Read the model definition and answer for the solid it produces. Units are mm, in the model's axes. Face numbers are marked on the shaded views. A direction names the side the tool comes from. Coordinates: 2 decimals unless noted, no trailing zeros. Write each loop counter-clockwise with the first axis right and the second up, starting at its lowest first coordinate (ties: lowest second). Pieces come first, ordered by that corner, then holes. Notation, with made-up numbers: (-0.75, 66) -> (20.25, 66) arc R26 ccw to (20.25, 87) -> close; hole circle Ø11 at (24.5, 5). An arc over 180 degrees is marked (long way). Answer in a Markdown table with one row per item. Add a question column.
Item 1: Given pin 1 Ø1 at (y, z) = (3.5, 31.5) entering from +X; pin 2 Ø4 at (y, z) = (-18, 16.5) entering from -X; pin 3 Ø16 at (x, y) = (-32.7, 0) entering from +Z, each flat-ended and moving along its own axis, determine where each tip first touches the part or whether it passes through.
Item 2: Which of the six approach directions +Z, -Z, +X, -X, +Y, -Y give full straight-line access (tool end or side, diameter ignored) to the marked faces 1 and 2?
Item 3: Section C-C on y = -15.5 is taken. Write down the section's boundary in (x, z), then the cut area to 3 significant figures.
Item 4: Section A-A on z = 5.5 is taken. Write down the section's boundary in (x, y), then the cut area to 3 significant figures.
Item 5: Section B-B on x = 12.5 is taken. Write down the section's boundary in (y, z).
Item 6: Straight lines are drawn through the part: line 1 (Y direction, x = 0, z = 36); line 2 (Y direction, x = 1, z = 12.5); line 3 (X direction, y = -3, z = 36). For each, find the intervals that lie inside material, in ascending order. Write a range as from..to.
Item 7: Section D-D on z = 23.5 is taken. Write down the section's boundary in (x, y), then the cut area to 3 significant figures.
Item 8: For a pull along Y with two mould halves and no side action, classify the marked faces 3, 4 and 5 as +Y half, -Y half, draft (parallel to the pull), parting line (faces both ways), or undercut.
```python
from build123d import *

# Parameters (mm, degrees)
F1_DEPTH = 20
F2_R     = 10
F3_R     = 25
F4_R     = 18
F5_DEPTH = 30
F7_D     = 10
F9_D     = 14
F9_DEPTH = 31
F9_TIP   = 4.2060243332


with BuildPart() as f1:
    # F0 (on Top) → F1 (new body)
    with BuildSketch(Plane.XY):
        Polygon((0, 27.6), (-55, 0), (0, -27.6), (55, 0), align=None)
    extrude(amount=F1_DEPTH)

    # F2
    f2_edges = [f1.edges().sort_by_distance(p)[0] for p in [
        (55, 0, 10),
        (-55, 0, 10),
    ]]
    fillet(f2_edges, radius=F2_R)

    # F3
    f3_edges = [f1.edges().sort_by_distance(p)[0] for p in [
        (0, -27.6, 10),
        (0, 27.6, 10),
    ]]
    fillet(f3_edges, radius=F3_R)

    # F4 (on face) → F5 (join)
    with BuildSketch(Plane.XY.offset(20)):
        Circle(F4_R)
    extrude(amount=F5_DEPTH)

    # F7 (through all)
    with Locations(Plane.XY.offset(20)):
        with Locations((-32.7041102381, 0), (32.7041102381, 0)):
            Hole(F7_D / 2)

    # F9
    with Locations(Plane.XY.offset(50)):
        with Locations((0, 0)):
            Hole(F9_D / 2, depth=F9_DEPTH)
            with Locations((0, 0, -(F9_DEPTH + F9_TIP / 2))):  # 118° drill point
                Cone(0, F9_D / 2, F9_TIP, mode=Mode.SUBTRACT)


solid = f1.part
```
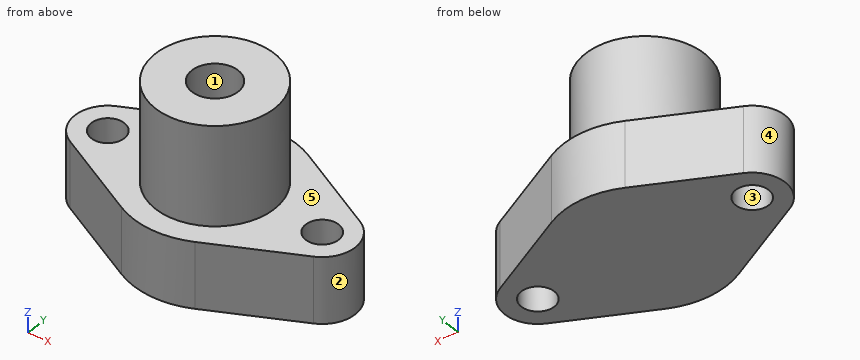
Results below:
| question | item | result |
|---|---|---|
| 1 | pin 1 | stops at x = 17.75 |
| 1 | pin 2 | stops at x = -23.12 |
| 1 | pin 3 | stops at z = 20 |
| 2 | face 1 | +Z |
| 2 | face 2 | +Z, -Z, +X |
| 3 | outline | (-24.11, 0) -> (24.11, 0) -> (24.11, 20) -> (9.15, 20) -> (9.15, 50) -> (-9.15, 50) -> (-9.15, 20) -> (-24.11, 20) -> close |
| 3 | area | 1,510 mm2 |
| 4 | outline | (-37.19, -8.94) -> (-11.21, -21.97) arc R25 ccw to (11.21, -21.97) -> (37.19, -8.94) arc R10 ccw to (37.19, 8.94) -> (11.21, 21.97) arc R25 ccw to (-11.21, 21.97) -> (-37.19, 8.94) arc R10 ccw to start; hole circle Ø10 at (-32.7, 0); hole circle Ø10 at (32.7, 0) |
| 4 | area | 2,660 mm2 |
| 5 | outline | (-21.33, 0) -> (21.33, 0) -> (21.33, 20) -> (12.95, 20) -> (12.95, 50) -> (-12.95, 50) -> (-12.95, 20) -> (-21.33, 20) -> close |
| 6 | line 1 | y = -18..-7, 7..18 |
| 6 | line 2 | y = -24.61..24.61 |
| 6 | line 3 | x = -17.75..-6.32, 6.32..17.75 |
| 7 | outline | circle Ø36 at (0, 0); hole circle Ø14 at (0, 0) |
| 7 | area | 864 mm2 |
| 8 | face 3 | undercut |
| 8 | face 4 | parting line |
| 8 | face 5 | draft |
